```python
from build123d import *

# Parameters (mm, degrees)
F0_W     = 120
F0_H     = 120
F0_R     = 5.5
F1_DEPTH = 6
F2_W     = 50
F2_H     = 50
F3_DEPTH = 750
F4_R     = 5


# Not quite as in the source:
# - a feature names something its author has since deleted; it is built from what else it names


with BuildPart() as f1:
    # F0 (on Top) → F1 (new body)
    with BuildSketch(Plane.XY):
        Rectangle(F0_W, F0_H)
        with Locations((-45, -45)):
            Circle(F0_R, mode=Mode.SUBTRACT)
        with Locations((45, -45)):
            Circle(F0_R, mode=Mode.SUBTRACT)
        with Locations((-45, 45)):
            Circle(F0_R, mode=Mode.SUBTRACT)
        with Locations((45, 45)):
            Circle(F0_R, mode=Mode.SUBTRACT)
    extrude(amount=F1_DEPTH)

    # F2 (on face) → F3 (join)
    with BuildSketch(Plane.XY.offset(6)):
        Rectangle(F2_W, F2_H)
    extrude(amount=F3_DEPTH)

    # F4
    f4_edges = [f1.edges().sort_by_distance(p)[0] for p in [
        (-25, -25, 381),
        (25, -25, 381),
        (25, 25, 381),
        (-25, 25, 381),
    ]]
    fillet(f4_edges, radius=F4_R)


solid = f1.part
```
Geometry: final body of the model. Coordinates: model frame, mm. A direction names the side the tool comes from. Round coordinates to 2 decimals unless told otherwise and drop trailing zeros. Order: outer loops, then holes, each group sorted by start corner. A loop starts at its lowest first (then second) coordinate and runs counter-clockwise, first axis right, second up. Notation, with made-up numbers: (61.5, -30) -> (93.5, -30) arc R28 ccw to (93.5, -12) -> close; hole circle Ø6 at (61, 46.5). An arc over 180 degrees is marked (long way). Use one line per item in the form item = value.
(1) Ray query, probe 1 along Y at (x, z) = (45, 2.35); probe 2 along Z at (x, y) = (-26.5, -5); probe 3 along X at (y, z) = (7.5, 558). Return the intervals inside material, ascending. Write a range as [from, to].
Results list:
probe_1 = [-60, -50.5], [-39.5, 39.5], [50.5, 60]
probe_2 = [0, 6]
probe_3 = [-25, 25]
(2) First-contact query: pin 1 Ø12 at (y, z) = (-7, 520) entering from +X; pin 2 Ø2 at (x, y) = (-46, -40.5) entering from +Z; pin 3 Ø3 at (x, y) = (43.5, 7) entering from -Z; pin 4 Ø12 at (x, z) = (-4.5, 287) entering from +Y. Flat tips, straight axial feed; report the tip coordinate or a pass-through.
Results list:
pin_1 = 25
pin_2 = 6
pin_3 = 0
pin_4 = 25
(3) Draft query along Z for faces 1 (the face through (25, 0, 376)), 2 (the face through (0, 0, 756)), 3 (the face through (-1, 1, 0)). Return one class per face: pulls with the +Z half, pulls with the -Z half, needs draft (parallel to the pull), parting line crosses it, or undercut.
Results list:
face_1 = needs draft
face_2 = pulls with the +Z half
face_3 = pulls with the -Z half
(4) Section B-B on z = 472. Return loops of the section in (x, y).
Results list:
outline = (-25, -20) arc R5 ccw to (-20, -25) -> (20, -25) arc R5 ccw to (25, -20) -> (25, 20) arc R5 ccw to (20, 25) -> (-20, 25) arc R5 ccw to (-25, 20) -> close
(5) Section A-A on y = -6. Return loops of the section in (x, z), and give its area (3 significant figures).
Results list:
outline = (-60, 0) -> (60, 0) -> (60, 6) -> (25, 6) -> (25, 756) -> (-25, 756) -> (-25, 6) -> (-60, 6) -> close
area = 38,200 mm^2
(6) Access query for faces 4 (the face through (0, -25, 376)), 5 (the face through (0, 25, 376)), 6 (the face through (-25, 0, 376)). Directions: +Z, -Z, +X, -X, +Y, -Y. A direction counts if a zero-diameter tool reaches every point of the face in a straight line with its end or side. Return the directions, or none.
Results list:
face_4 = +Z, +X, -X, -Y
face_5 = +Z, +X, -X, +Y
face_6 = +Z, -X, +Y, -Y
